from build123d import *

# Parameters (mm, degrees)
F1_DEPTH = 25.4
F2_DEPTH = 25.4
F3_DEPTH = 25.4


with BuildPart() as f1:
    # F0 (on Right) → F1 (new body)
    with BuildSketch(Plane.YZ):
        Polygon((-16.583575, 9.432823), (-16.488011, 9.432823), (17.062246, 9.432823), (17.15781, 9.432823), (17.062246, 14.338518), (-10.737195, 14.338518), align=None)
    extrude(amount=F1_DEPTH)

    # F0 (on Right) → F2 (join)
    with BuildSketch(Plane.YZ):
        with BuildLine():
            Line((-16.488011, 8.924823), (-14.59219, 8.924823))
            Line((-14.59219, 8.924823), (17.062246, 8.924823))
            ThreePointArc((17.062246, 8.924823), (17.12982, 8.952814), (17.15781, 9.020388))
            Line((17.15781, 9.020388), (17.15781, 9.337259))
            ThreePointArc((17.15781, 9.337259), (17.12982, 9.404833), (17.062246, 9.432823))
            Line((17.062246, 9.432823), (-16.488011, 9.432823))
            ThreePointArc((-16.488011, 9.432823), (-16.555585, 9.404833), (-16.583575, 9.337259))
            Line((-16.583575, 9.337259), (-16.583575, 9.020388))
            ThreePointArc((-16.583575, 9.020388), (-16.555585, 8.952814), (-16.488011, 8.924823))
        make_face()
    extrude(amount=F2_DEPTH)

    # F0 (on Right) → F3 (join)
    with BuildSketch(Plane.YZ):
        Polygon((17.062246, 8.924823), (-14.59219, 8.924823), (-14.59219, 5.485807), (-8.05446, 0), (-8.05446, -16.475177), (17.15781, -16.475177), (17.15781, 8.924823), align=None)
    extrude(amount=F3_DEPTH)


solid = f1.part
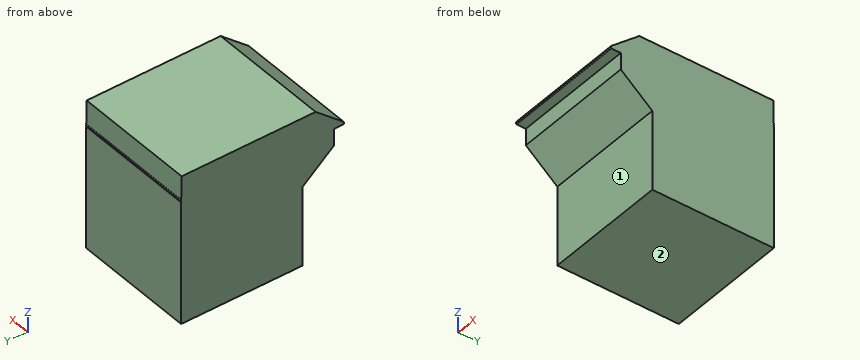
Input: part model. Units: mm. Frame: model coordinates. Face numbers are marked on the shaded views. A direction names the side the tool comes from. Coordinates: 2 decimals unless noted, no trailing zeros. Loops run counter-clockwise (first coordinate to the right, second up) from the corner with the lowest first, then second, coordinate; pieces in that order, holes last.
Q1. Contact query for flat-ended pins moving along their axis: pin 1 (4 mm diameter, centred on x = 5.5, z = -11, fed in from -Y); pin 2 (1.5 mm diameter, centred on x = 11.5, y = -15, fed in from -Z). Output: stop coordinate, or through.
Q2. Cut plane B-B (z = 8). Output: boundary loops of the cut face in (x, y).
Q3. Material intervals for line 1 (Y direction, x = 17.25, z = -5.5); line 2 (Y direction, x = 20.5, z = 9); line 3 (Z direction, x = 5, y = -13), sorted ascending.
Q4. Cut plane A-A (x = 9). Output: boundary loops of the cut face in (y, z).
Q5. Set-up query: the marked faces 1 and 2. Return all of +Z, -Z, +X, -X, +Y, -Y with unobstructed straight access to the full face (end or side cutting, diameter ignored); none if empty.
Q6. Cut plane C-C (y = -14). Output: boundary loops of the cut face in (x, z), then the cut area to 3 significant figures.
Working result:
1. pin 1: stops at y = -8.05
1. pin 2: stops at z = 5.2
2. outline: (0, -14.59) - (25.4, -14.59) - (25.4, 17.16) - (0, 17.16) - close
3. line 1: y = -8.05 to 17.16
3. line 2: y = -16.58 to 17.16
3. line 3: z = 4.15 to 12.44
4. outline: (-16.58, 9.02) arc R0.1 ccw to (-16.49, 8.92) - (-14.59, 8.92) - (-14.59, 5.49) - (-8.05, 0) - (-8.05, -16.48) - (17.16, -16.48) - (17.16, 8.92) - (17.06, 8.92) arc R0.1 ccw to (17.16, 9.02) - (17.16, 9.34) arc R0.1 ccw to (17.06, 9.43) - (17.16, 9.43) - (17.06, 14.34) - (-10.74, 14.34) - (-16.58, 9.43) - (-16.49, 9.43) arc R0.1 ccw to (-16.58, 9.34) - close
5. face 1: -Z, +X, -X, -Y
5. face 2: -Z, +X, -X, +Y, -Y
6. outline: (0, 4.99) - (25.4, 4.99) - (25.4, 11.6) - (0, 11.6) - close
6. area: 168 mm2
